Can you work these out from the model? Positions are in its coordinate system, mm. A direction names the side the tool comes from. Give positions to 0.01 mm unless a question says otherwise; leave off trailing zeros. Order: outer loops, then holes, each group sorted by start corner. A loop starts at its lowest first (then second) coordinate and runs counter-clockwise, first axis right, second up.
```python
from build123d import *

# Parameters (mm, degrees)
BOSS_EXTRUDE1_DEPTH             = 11.90625
FILLET1_R                       = 3.3782
FOR_CONNECTION_TO_DONUT_D       = 9.525
F_5_16_0_3125_DIAMETER_HOLE1_D  = 7.9375
CIRPATTERN1_COUNT               = 4
SKETCH14_R                      = 21.082
HOLE_FOR_WHEEL_ON_A_STICK_DEPTH = 342.457374776


with BuildPart() as part:
    # Sketch2 → Boss-Extrude1 (new body)
    with BuildSketch(Plane(origin=(0, 0, 0), x_dir=(1, 0, 0), z_dir=(0, 1, 0))):
        Polygon((-241.3, 241.3), (-139.7, 241.3), (-139.7, 207.9625), (139.7, 207.9625), (139.7, 241.3), (241.3, 241.3), (241.3, 139.7), (207.9625, 139.7), (207.9625, -139.7), (241.3, -139.7), (241.3, -241.3), (139.7, -241.3), (139.7, -207.9625), (-139.7, -207.9625), (-139.7, -241.3), (-241.3, -241.3), (-241.3, -139.7), (-207.9625, -139.7), (-207.9625, 139.7), (-241.3, 139.7), align=None)
    extrude(amount=-BOSS_EXTRUDE1_DEPTH)

    # Fillet1
    fillet1_edges = [part.edges().sort_by_distance(p)[0] for p in [
        (-139.7, -5.953125, -207.9625),
        (139.7, -5.953125, -207.9625),
        (207.9625, -5.953125, -139.7),
        (207.9625, -5.953125, 139.7),
        (139.7, -5.953125, 207.9625),
        (-139.7, -5.953125, 207.9625),
        (-207.9625, -5.953125, 139.7),
        (-207.9625, -5.953125, -139.7),
    ]]
    fillet(fillet1_edges, radius=FILLET1_R)

    # for connection to donut (through all)
    with Locations(Plane(origin=(0, -11.90625, 0), x_dir=(-1, 0, 0), z_dir=(0, -1, 0))):
        with Locations((0, -142.875), (142.875, 0), (0, 142.875), (-142.875, 0)):
            Hole(FOR_CONNECTION_TO_DONUT_D / 2)

    # 5/16 (0.3125) Diameter Hole1 (through all)
    with Locations(Plane(origin=(0, -11.90625, 0), x_dir=(-1, 0, 0), z_dir=(0, -1, 0))):
        with Locations((-157.1625, 201.6125), (-179.3875, 223.8375), (-223.8375, 179.3875), (-201.6125, 157.1625)):
            f_5_16_0_3125_diameter_hole1 = Hole(F_5_16_0_3125_DIAMETER_HOLE1_D / 2)

    # CirPattern1: 5/16 (0.3125) Diameter Hole1 ×4 about axis
    cirpattern1_axis = Axis((0, 0, 0), (0, 1, 0))
    for i in range(1, CIRPATTERN1_COUNT):
        add(f_5_16_0_3125_diameter_hole1.rotate(cirpattern1_axis, i * 360 / CIRPATTERN1_COUNT), mode=Mode.SUBTRACT)

    # Sketch14 → hole for wheel on a stick (cut, through all)
    with BuildSketch(Plane(origin=(0, 0, 0), x_dir=(1, 0, 0), z_dir=(0, 1, 0))):
        with Locations(Location((0, 0, 0), (0, 0, 270))):
            Circle(SKETCH14_R)
    extrude(amount=-HOLE_FOR_WHEEL_ON_A_STICK_DEPTH, mode=Mode.SUBTRACT)


solid = part.part
```
1) Suppose I cut it at C-C (y = -2.75). Give the number of separate pieces and of enclosed holes in the cut face, and give its area (3 significant figures).
2) I'm going to push flat-ended pins straight in: pin 1 Ø6 at (y, z) = (-3, -56.5) entering from +X; pin 2 Ø5.5 at (x, z) = (0, -142.875) entering from +Y; pin 3 Ø4 at (y, z) = (-3.5, -133) entering from -X; pin 4 Ø1 at (x, y) = (-93.5, -1.5) entering from -Z. Where does each tip first touch, or does it pass through?
3) Suppose I cut it at B-B (z = -64). Please give me the cut outline in (x, y), and give its area (3 significant figures).
4) If I drill on line 1 (Z direction, x = 132.5, y = -2.25); line 2 (X direction, y = -4, z = -15), over which ranges is the centre line in solid material (lowest first)?
5) Suppose I cut it at A-A (x = 79). Please give me the cut outline in (y, z), and give its area (3 significant figures).
6) We'd pull the mould along Z, two halves only. Please class faces 5 (the face through (227, -6, -139.7)), 6 (the face through (139.7, -6, 227)), 7 (the face through (190, -6, -241.3)): +Z half, -Z half, draft (parallel to the pull), parting line (faces both ways), or undercut.
7) Which directions (+Z, -Z, +X, -X, +Y, -Y) give clear straight access to the entire face, cutting with the end or side of a thin tool? Please do faces 1 (the face through (-207.962, -6, 2)), 2 (the face through (-2, -6, -207.962)), 3 (the face through (2, -6, 207.962)), 4 (the face through (207.962, -6, -2)).
Results:
1. separate pieces: 1
1. enclosed holes: 21
1. area: 193,000 mm2
2. pin 1: stops at x = 207.96
2. pin 2: passes through
2. pin 3: stops at x = -207.96
2. pin 4: stops at z = -207.96
3. outline: (-207.96, -11.91) - (207.96, -11.91) - (207.96, 0) - (-207.96, 0) - close
3. area: 4,950 mm2
4. line 1: z = -207.96 to 207.96
4. line 2: x = -207.96 to -14.81, 14.81 to 207.96
5. outline: (-11.91, -207.96) - (0, -207.96) - (0, 207.96) - (-11.91, 207.96) - close
5. area: 4,950 mm2
6. face 5: undercut
6. face 6: draft
6. face 7: -Z half
7. face 1: -X, +Y, -Y
7. face 2: -Z, +Y, -Y
7. face 3: +Z, +Y, -Y
7. face 4: +X, +Y, -Y
